Can you work these out from the model? Positions are in its coordinate system, mm. A direction names the side the tool comes from. Give positions to 0.01 mm unless a question says otherwise; leave off trailing zeros. Order: outer loops, then holes, each group sorted by start corner. A loop starts at its lowest first (then second) coordinate and runs counter-clockwise, first axis right, second up.
```python
from build123d import *

# Parameters (mm, degrees)
F0_W     = 76.2
F0_H     = 50.8
F0_R     = 12.7
F1_DEPTH = 12.7
F2_W     = 6.35
F2_H     = 50.8
F3_DEPTH = 2.54
F5_DEPTH = 50.8
F6_R     = 4.7625
F7_DEPTH = 12.7


with BuildPart() as f1:
    # F0 (on Top) → F1 (new body)
    with BuildSketch(Plane.XY):
        with Locations((1.190625, 0)):
            Rectangle(F0_W, F0_H)
        Circle(F0_R, mode=Mode.SUBTRACT)
    extrude(amount=F1_DEPTH)

    # F2 (on face) → F3 (cut)
    with BuildSketch(Plane.XY.offset(12.7)):
        with Locations((-31.194375, 0)):
            Rectangle(F2_W, F2_H)
        with BuildLine():
            Line((-6.35, -10.9985226281), (-6.35, -25.4))
            Line((-6.35, -25.4), (6.35, -25.4))
            Line((6.35, -25.4), (6.35, -10.9985226281))
            ThreePointArc((6.35, -10.9985226281), (0, -12.7), (-6.35, -10.9985226281))
        make_face()
        with BuildLine():
            Line((6.35, 25.4), (-6.35, 25.4))
            Line((-6.35, 25.4), (-6.35, 10.9985226281))
            ThreePointArc((-6.35, 10.9985226281), (0, 12.7), (6.35, 10.9985226281))
            Line((6.35, 10.9985226281), (6.35, 25.4))
        make_face()
    extrude(amount=-F3_DEPTH, mode=Mode.SUBTRACT)

    # F4 (on face) → F5 (cut)
    with BuildSketch(Plane.XZ.offset(25.4)):
        Polygon((31.75, 12.7), (19.05, 12.7), (16.1170606325, 7.62), (34.6829393675, 7.62), align=None)
    extrude(amount=-F5_DEPTH, mode=Mode.SUBTRACT)

    # F6 (on face) → F7 (join)
    with BuildSketch(Plane.YZ.offset(39.290625)):
        with Locations((0, 6.35)):
            Circle(F6_R)
    extrude(amount=F7_DEPTH)


solid = f1.part
```
1) If I drill on line 1 (X direction, y = 0, z = 6.75); line 2 (Y direction, x = 0, z = 3.75); line 3 (X direction, y = -9, z = 11), over which ranges is the centre line in solid material (lowest first)?
2) I'm going to push flat-ended pins straight in: pin 1 Ø3 at (y, z) = (-12.5, 11.5) entering from +X; pin 2 Ø1.9 at (x, y) = (-32, 9) entering from +Z. Where does each tip first touch, or does it pass through?
3) Suppose I cut it at C-C (z = 6.35). Please give me the cut outline in (x, y), and give its area (3 significant figures).
4) Which directions (+Z, -Z, +X, -X, +Y, -Y) give clear straight access to the entire face, cutting with the end or side of a thin tool? Please do faces 1 (the face through (14, 0, 12.7)), 2 (the face through (-6.35, 18, 11)), 3 (the face through (25, 0, 7.62)).
5) Suppose I cut it at B-B (x = 0). Please give me the cut outline in (y, z), and give its area (3 significant figures).
6) Suppose I cut it at A-A (y = 0). Please give me the cut outline in (x, z).
7) We'd pull the mould along X, two halves only. Please class faces 4 (the face through (45.55, -1.03, 1.7)), 5 (the face through (51.991, 0, 6)), 6 (the face through (-1.653, 12.592, 6.261)), 7 (the face through (17.604, -0.356, 10.196)): +X half, -X half, draft (parallel to the pull), parting line (faces both ways), or undercut.
8) Suppose I cut it at D-D (y = 15). Please give me the cut outline in (x, z).
Results:
1. line 1: x = -36.91 to -12.7, 12.7 to 51.99
1. line 2: y = -25.4 to -12.7, 12.7 to 25.4
1. line 3: x = -36.91 to -34.37, -28.02 to -8.96, 8.96 to 18.07, 32.73 to 39.29
2. pin 1: stops at x = 39.29
2. pin 2: stops at z = 10.16
3. outline: (-36.91, -25.4) - (39.29, -25.4) - (39.29, -4.76) - (51.99, -4.76) - (51.99, 4.76) - (39.29, 4.76) - (39.29, 25.4) - (-36.91, 25.4) - close; hole circle Ø25.4 at (0, 0)
3. area: 3,490 mm2
4. face 1: +Z, +X, -X, +Y, -Y
4. face 2: +Z, +Y, -Y
4. face 3: +Y, -Y
5. outline: (-25.4, 0) - (-12.7, 0) - (-12.7, 10.16) - (-25.4, 10.16) - close; (12.7, 0) - (25.4, 0) - (25.4, 10.16) - (12.7, 10.16) - close
5. area: 258 mm2
6. outline: (-36.91, 0) - (-12.7, 0) - (-12.7, 12.7) - (-28.02, 12.7) - (-28.02, 10.16) - (-34.37, 10.16) - (-34.37, 12.7) - (-36.91, 12.7) - close; (12.7, 0) - (39.29, 0) - (39.29, 1.59) - (51.99, 1.59) - (51.99, 11.11) - (39.29, 11.11) - (39.29, 12.7) - (31.75, 12.7) - (34.68, 7.62) - (16.12, 7.62) - (19.05, 12.7) - (12.7, 12.7) - close
7. face 4: draft
7. face 5: +X half
7. face 6: undercut
7. face 7: undercut
8. outline: (-36.91, 0) - (39.29, 0) - (39.29, 12.7) - (31.75, 12.7) - (34.68, 7.62) - (16.12, 7.62) - (19.05, 12.7) - (6.35, 12.7) - (6.35, 10.16) - (-6.35, 10.16) - (-6.35, 12.7) - (-28.02, 12.7) - (-28.02, 10.16) - (-34.37, 10.16) - (-34.37, 12.7) - (-36.91, 12.7) - close
